```python
from build123d import *

# Parameters (mm, degrees)
SKETCH_1_W          = 95
SKETCH_1_H          = 68
EXTRUDE_1_DEPTH     = 7.5
CUT_EXTRUDE_1_DEPTH = 6.5
SKETCH_3_W          = 77
SKETCH_3_H          = 52
CUT_EXTRUDE_2_DEPTH = 59.893972527
SKETCH_4_R          = 2.1
CUT_EXTRUDE_3_DEPTH = 2.6
FILLET_1_R          = 1
FILLET_2_R          = 1


with BuildPart() as part:
    # 草图1 → 凸台-拉伸1 (new body)
    with BuildSketch(Plane(origin=(0, 0, 0), x_dir=(1, 0, 0), z_dir=(0, 1, 0))):
        Rectangle(SKETCH_1_W, SKETCH_1_H)
    extrude(amount=EXTRUDE_1_DEPTH)

    # 草图2 → 切除-拉伸1 (cut)
    with BuildSketch(Plane.XZ):
        Polygon((-45.5, 28.1), (40.5, 28.1), (40.5, -28.1), (-45.5, -28.1), (-45.5, -18), (-46, -18), (-46, 25), (-45.5, 25), align=None)
    extrude(amount=-CUT_EXTRUDE_1_DEPTH, mode=Mode.SUBTRACT)

    # 草图3 → 切除-拉伸2 (cut, through all)
    with BuildSketch(Plane(origin=(0, 7.5, 0), x_dir=(1, 0, 0), z_dir=(0, 1, 0))):
        Rectangle(SKETCH_3_W, SKETCH_3_H)
    extrude(amount=-CUT_EXTRUDE_2_DEPTH, mode=Mode.SUBTRACT)

    # 草图4 → 切除-拉伸3 (cut)
    with BuildSketch(Plane.XZ):
        with Locations(Location((-44.5, 31, 0), (0, 0, 270))):
            Circle(SKETCH_4_R)
        with Locations(Location((0, 31, 0), (0, 0, 270))):
            Circle(SKETCH_4_R)
        with Locations(Location((44.5, 31, 0), (0, 0, 270))):
            Circle(SKETCH_4_R)
        with Locations(Location((44.5, -31, 0), (0, 0, 270))):
            Circle(SKETCH_4_R)
        with Locations(Location((0, -31, 0), (0, 0, 270))):
            Circle(SKETCH_4_R)
        with Locations(Location((-44.5, -31, 0), (0, 0, 270))):
            Circle(SKETCH_4_R)
    extrude(amount=-CUT_EXTRUDE_3_DEPTH, mode=Mode.SUBTRACT)

    # 圆角1
    fillet_1_edges = [part.edges().sort_by_distance(p)[0] for p in [
        (-47.5, 7.5, 0),
        (0, 7.5, 34),
        (47.5, 7.5, 0),
        (0, 7.5, -34),
    ]]
    fillet(fillet_1_edges, radius=FILLET_1_R)

    # 圆角2
    # the kernel refuses this fillet: 1 mm, written as the material it takes off along each edge
    with BuildSketch(Plane(origin=(46.5, 6.5, -33), x_dir=(0, 0, -1), z_dir=(1, 0, 0))) as fillet_2_piece_1_section:
        Polygon((0, 0), (FILLET_2_R, 0), (FILLET_2_R, FILLET_2_R), (0, FILLET_2_R), align=None)
    fillet_2_piece_1 = extrude(amount=FILLET_2_R, mode=Mode.PRIVATE)
    fillet_2_piece_1 = fillet_2_piece_1 - Plane(origin=(46.5, 6.5, -33), x_dir=(0, -0.7071067811865475, 0.7071067811865475), z_dir=(1, 0, 0)) * Sphere(FILLET_2_R, mode=Mode.PRIVATE)
    add(fillet_2_piece_1, mode=Mode.SUBTRACT)
    with BuildSketch(Plane(origin=(46.5, 6.5, 33), x_dir=(1, 0, 0), z_dir=(0, 0, 1))) as fillet_2_piece_2_section:
        Polygon((0, 0), (FILLET_2_R, 0), (FILLET_2_R, FILLET_2_R), (0, FILLET_2_R), align=None)
    fillet_2_piece_2 = extrude(amount=FILLET_2_R, mode=Mode.PRIVATE)
    fillet_2_piece_2 = fillet_2_piece_2 - Plane(origin=(46.5, 6.5, 33), x_dir=(-0.7071067811865475, -0.7071067811865475, 0), z_dir=(0, 0, 1)) * Sphere(FILLET_2_R, mode=Mode.PRIVATE)
    add(fillet_2_piece_2, mode=Mode.SUBTRACT)
    with BuildSketch(Plane(origin=(-46.5, 6.5, -33), x_dir=(0, 0, -1), z_dir=(-1, 0, 0))) as fillet_2_piece_3_section:
        Polygon((0, 0), (FILLET_2_R, 0), (FILLET_2_R, -FILLET_2_R), (0, -FILLET_2_R), align=None)
    fillet_2_piece_3 = extrude(amount=FILLET_2_R, mode=Mode.PRIVATE)
    fillet_2_piece_3 = fillet_2_piece_3 - Plane(origin=(-46.5, 6.5, -33), x_dir=(0, -0.7071067811865475, 0.7071067811865475), z_dir=(-1, 0, 0)) * Sphere(FILLET_2_R, mode=Mode.PRIVATE)
    add(fillet_2_piece_3, mode=Mode.SUBTRACT)
    with BuildSketch(Plane(origin=(-46.5, 6.5, 33), x_dir=(-1, 0, 0), z_dir=(0, 0, 1))) as fillet_2_piece_4_section:
        Polygon((0, 0), (FILLET_2_R, 0), (FILLET_2_R, -FILLET_2_R), (0, -FILLET_2_R), align=None)
    fillet_2_piece_4 = extrude(amount=FILLET_2_R, mode=Mode.PRIVATE)
    fillet_2_piece_4 = fillet_2_piece_4 - Plane(origin=(-46.5, 6.5, 33), x_dir=(0.7071067811865475, -0.7071067811865475, 0), z_dir=(0, 0, 1)) * Sphere(FILLET_2_R, mode=Mode.PRIVATE)
    add(fillet_2_piece_4, mode=Mode.SUBTRACT)
    with BuildSketch(Plane(origin=(-47.5, -2.5, 34), x_dir=(1, 0, 0), z_dir=(0, 1, 0)), Plane(origin=(-47.5, -2.5, -34), x_dir=(0, 0, 1), z_dir=(0, 1, 0))) as fillet_2_piece_5:
        with BuildLine():
            CenterArc((FILLET_2_R, FILLET_2_R), FILLET_2_R, 180, 90)
            Line((0, FILLET_2_R), (0, 0))
            Line((0, 0), (FILLET_2_R, 0))
        make_face()
    extrude(amount=9, mode=Mode.SUBTRACT)
    with BuildSketch(Plane(origin=(47.5, -2.5, -34), x_dir=(0, 0, 1), z_dir=(0, 1, 0)), Plane(origin=(47.5, -2.5, 34), x_dir=(-1, 0, 0), z_dir=(0, 1, 0))) as fillet_2_piece_6:
        with BuildLine():
            CenterArc((FILLET_2_R, -FILLET_2_R), FILLET_2_R, 90, 90)
            Line((0, -FILLET_2_R), (0, 0))
            Line((0, 0), (FILLET_2_R, 0))
        make_face()
    extrude(amount=9, mode=Mode.SUBTRACT)


solid = part.part
```
Source: CAD feature listing. Evaluate the final solid. Frame: model axes, mm. A direction names the side the tool comes from. Round coordinates to 2 decimals unless told otherwise and drop trailing zeros. Loops run counter-clockwise (first coordinate to the right, second up) from the corner with the lowest first, then second, coordinate; pieces in that order, holes last. Notation, with made-up numbers: M 75.25,38.25 L 129.25,38.25 A20 cw 129.25,73.25 Z; hole C 26.5,77.5 d3. An arc over 180 degrees is marked long. Put each result on its own line as item: value.
(1) First-contact query: pin 1 (4 mm diameter, centred on x = -44.5, z = 31, fed in from -Y); pin 2 (0.5 mm diameter, centred on x = -11.5, y = 7, fed in from -Z). Flat tips, straight axial feed; report the tip coordinate or a pass-through.
Solutions:
pin 1: y = 2.6
pin 2: z = -33.97
(2) Pull-direction query (X, two-part tool) for faces 1 (the face through (-46, 3, 3)), 2 (the face through (-47.5, 3, 0)), 3 (the face through (-12, 6.5, -27)), 4 (the face through (-1, 3, -34)); classes: released by +X, released by -X, zero draft, split by the parting line, or undercut.
Solutions:
face 1: undercut
face 2: released by -X
face 3: undercut
face 4: zero draft
(3) Access query for faces 5 (the face through (0, 2.6, 31)), 6 (the face through (10, 0, 30)). Directions: +Z, -Z, +X, -X, +Y, -Y. A direction counts if a zero-diameter tool reaches every point of the face in a straight line with its end or side. Return the directions, or none.
Solutions:
face 5: -Y
face 6: +Z, -Z, +X, -X, -Y
(4) Section D-D, the plane x = 44.5. Return loops of the section in (y, z), and give its area (3 significant figures).
Solutions:
outline: M 0,-34 L 6.5,-34 A1 ccw 7.5,-33 L 7.5,33 A1 ccw 6.5,34 L 0,34 L 0,33.1 L 2.6,33.1 L 2.6,28.9 L 0,28.9 L 0,-28.9 L 2.6,-28.9 L 2.6,-33.1 L 0,-33.1 Z
area: 488 mm²
(5) Section B-B, the plane x = -23. Return loops of the section in (y, z), and give its area (3 significant figures).
Solutions:
outline: M 0,-34 L 6.5,-34 A1 ccw 7.5,-33 L 7.5,-26 L 6.5,-26 L 6.5,-28.1 L 0,-28.1 Z; M 0,28.1 L 6.5,28.1 L 6.5,26 L 7.5,26 L 7.5,33 A1 ccw 6.5,34 L 0,34 Z
area: 92.3 mm²
(6) Section A-A, the plane z = -9. Return loops of the section in (x, y), and give its area (3 significant figures).
Solutions:
outline: M -47.5,0 L -46,0 L -46,6.5 L -38.5,6.5 L -38.5,7.5 L -46.5,7.5 A1 ccw -47.5,6.5 Z; M 38.5,6.5 L 40.5,6.5 L 40.5,0 L 47.5,0 L 47.5,6.5 A1 ccw 46.5,7.5 L 38.5,7.5 Z
area: 72.8 mm²
(7) Ray query, line 1 (X direction, y = 1.1, z = -31); line 2 (Z direction, x = -39, y = 1.5); line 3 (X direction, y = 5.75, z = 24). Return the intervals inside material, ascending. Write a range as [from, to].
Solutions:
line 1: [-47.5, -46.6], [-42.4, -2.1], [2.1, 42.4], [46.6, 47.5]
line 2: [-34, -28.1], [28.1, 34]
line 3: [-47.5, -46], [40.5, 47.5]
(8) Section C-C, the plane y = 4.25. Return loops of the section in (x, z), and give its area (3 significant figures).
Solutions:
outline: M -47.5,-33 A1 ccw -46.5,-34 L 46.5,-34 A1 ccw 47.5,-33 L 47.5,33 A1 ccw 46.5,34 L -46.5,34 A1 ccw -47.5,33 Z; hole M -46,-18 L -45.5,-18 L -45.5,-28.1 L 40.5,-28.1 L 40.5,28.1 L -45.5,28.1 L -45.5,25 L -46,25 Z
area: 1,600 mm²
